from build123d import *

# Parameters (mm, degrees)
SKETCH1_W           = 1200
SKETCH1_H           = 600
BOSS_EXTRUDE1_DEPTH = 25
SKETCH2_R           = 15
BOSS_EXTRUDE2_DEPTH = 725
CHAMFER1_SIZE       = 2


with BuildPart() as part:
    # Sketch1 → Boss-Extrude1 (new body)
    with BuildSketch(Plane.XY):
        Rectangle(SKETCH1_W, SKETCH1_H)
    extrude(amount=BOSS_EXTRUDE1_DEPTH)

    # Sketch2 → Boss-Extrude2 (add)
    with BuildSketch(Plane.XY):
        with Locations((550, 250)):
            Circle(SKETCH2_R)
        with Locations((-550, 250)):
            Circle(SKETCH2_R)
        with Locations((-550, -250)):
            Circle(SKETCH2_R)
        with Locations((550, -250)):
            Circle(SKETCH2_R)
    extrude(amount=-BOSS_EXTRUDE2_DEPTH)

    # Chamfer1
    chamfer1_edges = [part.edges().sort_by_distance(p)[0] for p in [
        (-600, 0, 25),
        (0, -300, 25),
        (600, 0, 25),
        (0, 300, 25),
    ]]
    chamfer(chamfer1_edges, length=CHAMFER1_SIZE)


solid = part.part
Geometry: final body of the model. Coordinates: model frame, mm. A direction names the side the tool comes from. Give positions to 0.01 mm unless a question says otherwise; leave off trailing zeros. Write each loop counter-clockwise with the first axis right and the second up, starting at its lowest first coordinate (ties: lowest second). Pieces come first, ordered by that corner, then holes. Notation, with made-up numbers: M 25,-23.75 L 56,-23.75 A12 ccw 56,-7.75 Z; hole C 39,63 d5. An arc over 180 degrees is marked long. Answer in a Markdown table with one row per item. Add a question column.
(1) Ray query, line 1 (X direction, y = 248.5, z = -542); line 2 (Z direction, x = -361.5, y = 209.5); line 3 (X direction, y = -258.5, z = -512.5). Return the intervals inside material, ascending.
(2) Section B-B on z = -396.5. Return loops of the section in (x, y), and give its area (3 significant figures).
(3) Section A-A on x = -550. Return loops of the section in (y, z).
(4) First-contact query: pin 1 (4 mm diameter, centred on x = 468.5, y = 144, fed in from -Z). Flat tip, straight axial feed; report the tip coordinate or a pass-through.
(5) Section C-C on y = -250. Return loops of the section in (x, z), and give its area (3 significant figures).
(6) Reachability of faces 3 (the cylindrical face through (-536.144, -255.745, -357.425)), 4 (the flat face through (550, -250, -725)) from +Z, -Z, +X, -X, +Y, -Y: full face, straight path, thin tool, end or side. Return the list, or none.
(7) Mould query, pull axis X, two halves, no side actions, for faces 1 (the flat face through (550, 250, -725)), 2 (the cylindrical face through (563.856, -255.745, -357.425)). Classes: +X half, -X half, draft (parallel to the pull), parting line (faces both ways), or undercut.
Result set:
| question | item | result |
|---|---|---|
| 1 | line 1 | x = -564.92 to -535.08, 535.08 to 564.92 |
| 1 | line 2 | z = 0 to 25 |
| 1 | line 3 | x = -562.36 to -537.64, 537.64 to 562.36 |
| 2 | outline | C -550,-250 d30; C -550,250 d30; C 550,-250 d30; C 550,250 d30 |
| 2 | area | 2,830 mm^2 |
| 3 | outline | M -300,0 L -265,0 L -265,-725 L -235,-725 L -235,0 L 235,0 L 235,-725 L 265,-725 L 265,0 L 300,0 L 300,23 L 298,25 L -298,25 L -300,23 Z |
| 4 | pin 1 | stops at z = 0 |
| 5 | outline | M -600,0 L -565,0 L -565,-725 L -535,-725 L -535,0 L 535,0 L 535,-725 L 565,-725 L 565,0 L 600,0 L 600,23 L 598,25 L -598,25 L -600,23 Z |
| 5 | area | 73,500 mm^2 |
| 6 | face 3 | -Z |
| 6 | face 4 | -Z, +X, -X, +Y, -Y |
| 7 | face 1 | draft |
| 7 | face 2 | undercut |
